```python
from build123d import *

# Parameters (mm, degrees)
SKETCH_3_W                      = 27
SKETCH_3_H                      = 27
EXTRUDE_1_DEPTH                 = 3
FILLET_1_R                      = 2
SKETCH_4_R                      = 1.1
CUT_EXTRUDE_1_DEPTH             = 6
SKETCH_5_R                      = 1.55
CUT_EXTRUDE_2_DEPTH             = 6
SKETCH_6_R                      = 1.05
CUT_EXTRUDE_3_DEPTH             = 6
PATTERN_CIRCULAR_1_COUNT        = 4
SKETCH_7_R                      = 4
CUT_EXTRUDE_4_DEPTH             = 1
CUT_EXTRUDE_8_DEPTH             = 21.012496096
PATTERN_CIRCULAR_2_COUNT        = 4
PATTERN_CIRCULAR_2_COPY_1_DEPTH = 21.012496096
PATTERN_CIRCULAR_2_COPY_2_DEPTH = 21.012496096
PATTERN_CIRCULAR_2_COPY_3_DEPTH = 21.012496096
SKETCH_12_R                     = 1.35
CUT_EXTRUDE_9_DEPTH             = 8
PATTERN_CIRCULAR_3_COUNT        = 4
EXTRUDE_2_DEPTH                 = 0.75
PATTERN_CIRCULAR_4_COUNT        = 4
PATTERN_CIRCULAR_4_COPY_1_DEPTH = 0.75
PATTERN_CIRCULAR_4_COPY_2_DEPTH = 0.75
PATTERN_CIRCULAR_4_COPY_3_DEPTH = 0.75
SKETCH_22_W                     = 2.7
SKETCH_22_H                     = 3
CUT_EXTRUDE_15_DEPTH            = 2
PATTERN_CIRCULAR_11_COUNT       = 4
SKETCH_31_W                     = 88
SKETCH_31_H                     = 100
EXTRUDE_4_DEPTH                 = 18
SKETCH_32_W                     = 78
SKETCH_32_H                     = 8.5
CUT_EXTRUDE_17_DEPTH            = 95


with BuildPart() as part:
    # ｽｹｯﾁ3 → ﾎﾞｽ - 押し出し1 (new, symmetric)
    with BuildSketch(Plane(origin=(0, 0, 0), x_dir=(1, 0, 0), z_dir=(0, 1, 0))):
        Rectangle(SKETCH_3_W, SKETCH_3_H)
    extrude(amount=EXTRUDE_1_DEPTH, both=True)

    # ﾌｨﾚｯﾄ1
    fillet_1_edges = [part.edges().sort_by_distance(p)[0] for p in [
        (13.5, 0, 13.5),
        (-13.5, 0, 13.5),
        (-13.5, 0, -13.5),
        (13.5, 0, -13.5),
    ]]
    fillet(fillet_1_edges, radius=FILLET_1_R)

    # ｽｹｯﾁ4 → ｶｯﾄ - 押し出し1 (cut)
    with BuildSketch(Plane(origin=(0, 3, 0), x_dir=(1, 0, 0), z_dir=(0, 1, 0))):
        with Locations(Location((-10.5, 10.5, 0), (0, 0, 270))):
            Circle(SKETCH_4_R)
        with Locations(Location((10.5, 10.5, 0), (0, 0, 270))):
            Circle(SKETCH_4_R)
        with Locations(Location((-10.5, -10.5, 0), (0, 0, 270))):
            Circle(SKETCH_4_R)
        with Locations(Location((10.5, -10.5, 0), (0, 0, 270))):
            Circle(SKETCH_4_R)
    extrude(amount=-CUT_EXTRUDE_1_DEPTH, mode=Mode.SUBTRACT)

    # ｽｹｯﾁ5 → ｶｯﾄ - 押し出し2 (cut)
    with BuildSketch(Plane(origin=(0, 3, 0), x_dir=(1, 0, 0), z_dir=(0, 1, 0))):
        with Locations(Location((0, 0, 0), (0, 0, 270))):
            Circle(SKETCH_5_R)
    extrude(amount=-CUT_EXTRUDE_2_DEPTH, mode=Mode.SUBTRACT)

    # ｽｹｯﾁ6 → ｶｯﾄ - 押し出し3 (cut)
    with BuildSketch(Plane(origin=(0, 3, 0), x_dir=(1, 0, 0), z_dir=(0, 1, 0))):
        with Locations(Location((4.242640687, 4.242640687, 0), (0, 0, 270))):
            Circle(SKETCH_6_R)
    cut_extrude_3 = extrude(amount=-CUT_EXTRUDE_3_DEPTH, mode=Mode.SUBTRACT)

    # 円形ﾊﾟﾀｰﾝ1: ｶｯﾄ - 押し出し3 ×4 about axis
    pattern_circular_1_axis = Axis((0, 0, 0), (0, 1, 0))
    for i in range(1, PATTERN_CIRCULAR_1_COUNT):
        add(cut_extrude_3.rotate(pattern_circular_1_axis, i * 360 / PATTERN_CIRCULAR_1_COUNT), mode=Mode.SUBTRACT)

    # ｽｹｯﾁ7 → ｶｯﾄ - 押し出し4 (cut)
    with BuildSketch(Plane(origin=(0, 3, 0), x_dir=(1, 0, 0), z_dir=(0, 1, 0))):
        with Locations(Location((0, 0, 0), (0, 0, 270))):
            Circle(SKETCH_7_R)
    extrude(amount=-CUT_EXTRUDE_4_DEPTH, mode=Mode.SUBTRACT)

    # ｽｹｯﾁ11 → ｶｯﾄ - 押し出し8 (cut, symmetric)
    with BuildSketch(Plane(origin=(0, 3, 0), x_dir=(1, 0, 0), z_dir=(0, 1, 0))):
        Polygon((-28.082033535, 86.024744916), (3, 13.5), (4.5, 10), (7, 10), (7.9, 13.5), (27.55047658, 89.918520033), (16.532211377, 247.342544779), (-39.100298738, 243.448769662), align=None)
    cut_extrude_8 = extrude(amount=CUT_EXTRUDE_8_DEPTH, both=True, mode=Mode.SUBTRACT)

    # ﾐﾗｰ1: ｶｯﾄ - 押し出し8 across plane
    add(cut_extrude_8.mirror(Plane(origin=(0, 0, 0), x_dir=(0, 0, 1), z_dir=(1, 0, 0))), mode=Mode.SUBTRACT)

    # 円形ﾊﾟﾀｰﾝ2: ｶｯﾄ - 押し出し8 ×4 about axis
    pattern_circular_2_axis = Axis((0, 0, 0), (0, 1, 0))
    for i in range(1, PATTERN_CIRCULAR_2_COUNT):
        add(cut_extrude_8.rotate(pattern_circular_2_axis, i * 360 / PATTERN_CIRCULAR_2_COUNT), mode=Mode.SUBTRACT)

    # 円形ﾊﾟﾀｰﾝ2 copy 1 sketch → 円形ﾊﾟﾀｰﾝ2 copy 1 (cut, symmetric)
    with BuildSketch(Plane.ZX.offset(3)):
        Polygon((-28.082033535, -86.024744916), (3, -13.5), (4.5, -10), (7, -10), (7.9, -13.5), (27.55047658, -89.918520033), (16.532211377, -247.342544779), (-39.100298738, -243.448769662), align=None)
    extrude(amount=PATTERN_CIRCULAR_2_COPY_1_DEPTH, both=True, mode=Mode.SUBTRACT)

    # 円形ﾊﾟﾀｰﾝ2 copy 2 sketch → 円形ﾊﾟﾀｰﾝ2 copy 2 (cut, symmetric)
    with BuildSketch(Plane(origin=(0, 3, 0), x_dir=(1, 0, 0), z_dir=(0, 1, 0))):
        Polygon((-28.082033535, -86.024744916), (3, -13.5), (4.5, -10), (7, -10), (7.9, -13.5), (27.55047658, -89.918520033), (16.532211377, -247.342544779), (-39.100298738, -243.448769662), align=None)
    extrude(amount=PATTERN_CIRCULAR_2_COPY_2_DEPTH, both=True, mode=Mode.SUBTRACT)

    # 円形ﾊﾟﾀｰﾝ2 copy 3 sketch → 円形ﾊﾟﾀｰﾝ2 copy 3 (cut, symmetric)
    with BuildSketch(Plane(origin=(0, 3, 0), x_dir=(0, 0, -1), z_dir=(0, 1, 0))):
        Polygon((-28.082033535, -86.024744916), (3, -13.5), (4.5, -10), (7, -10), (7.9, -13.5), (27.55047658, -89.918520033), (16.532211377, -247.342544779), (-39.100298738, -243.448769662), align=None)
    extrude(amount=PATTERN_CIRCULAR_2_COPY_3_DEPTH, both=True, mode=Mode.SUBTRACT)

    # ｽｹｯﾁ12 → ｶｯﾄ - 押し出し9 (cut)
    with BuildSketch(Plane.XY.offset(13.5)):
        Circle(SKETCH_12_R)
    cut_extrude_9 = extrude(amount=-CUT_EXTRUDE_9_DEPTH, mode=Mode.SUBTRACT)

    # 円形ﾊﾟﾀｰﾝ3: ｶｯﾄ - 押し出し9 ×4 about axis
    pattern_circular_3_axis = Axis((0, 0, 0), (0, 1, 0))
    for i in range(1, PATTERN_CIRCULAR_3_COUNT):
        add(cut_extrude_9.rotate(pattern_circular_3_axis, i * 360 / PATTERN_CIRCULAR_3_COUNT), mode=Mode.SUBTRACT)

    # ｽｹｯﾁ13 → ﾎﾞｽ - 押し出し2 (add, symmetric)
    with BuildSketch(Plane(origin=(0, 0, 0), x_dir=(1, 0, 0), z_dir=(0, 1, 0))):
        Polygon((7.9, 13.5), (7, 10), (6.5, 10), (7.4, 13.5), align=None)
        Polygon((3, 13.5), (3.5, 13.5), (5, 10), (4.5, 10), align=None)
    extrude_2 = extrude(amount=EXTRUDE_2_DEPTH, both=True)

    # ﾐﾗｰ2: ﾎﾞｽ - 押し出し2 across plane
    add(extrude_2.mirror(Plane(origin=(0, 0, 0), x_dir=(0, 0, 1), z_dir=(1, 0, 0))))

    # 円形ﾊﾟﾀｰﾝ4: ﾎﾞｽ - 押し出し2 ×4 about axis
    pattern_circular_4_axis = Axis((0, 0, 0), (0, 1, 0))
    for i in range(1, PATTERN_CIRCULAR_4_COUNT):
        add(extrude_2.rotate(pattern_circular_4_axis, i * 360 / PATTERN_CIRCULAR_4_COUNT))

    # 円形ﾊﾟﾀｰﾝ4 copy 1 sketch → 円形ﾊﾟﾀｰﾝ4 copy 1 (add, symmetric)
    with BuildSketch(Plane.ZX):
        Polygon((7.9, -13.5), (7, -10), (6.5, -10), (7.4, -13.5), align=None)
        Polygon((3, -13.5), (3.5, -13.5), (5, -10), (4.5, -10), align=None)
    extrude(amount=PATTERN_CIRCULAR_4_COPY_1_DEPTH, both=True)

    # 円形ﾊﾟﾀｰﾝ4 copy 2 sketch → 円形ﾊﾟﾀｰﾝ4 copy 2 (add, symmetric)
    with BuildSketch(Plane(origin=(0, 0, 0), x_dir=(1, 0, 0), z_dir=(0, 1, 0))):
        Polygon((7.9, -13.5), (7, -10), (6.5, -10), (7.4, -13.5), align=None)
        Polygon((3, -13.5), (3.5, -13.5), (5, -10), (4.5, -10), align=None)
    extrude(amount=PATTERN_CIRCULAR_4_COPY_2_DEPTH, both=True)

    # 円形ﾊﾟﾀｰﾝ4 copy 3 sketch → 円形ﾊﾟﾀｰﾝ4 copy 3 (add, symmetric)
    with BuildSketch(Plane(origin=(0, 0, 0), x_dir=(0, 0, -1), z_dir=(0, 1, 0))):
        Polygon((7.9, -13.5), (7, -10), (6.5, -10), (7.4, -13.5), align=None)
        Polygon((3, -13.5), (3.5, -13.5), (5, -10), (4.5, -10), align=None)
    extrude(amount=PATTERN_CIRCULAR_4_COPY_3_DEPTH, both=True)

    # ｽｹｯﾁ22 → ｶｯﾄ - 押し出し15 (cut)
    with BuildSketch(Plane.XY.offset(13.5)):
        with Locations((0, 1.5)):
            Rectangle(SKETCH_22_W, SKETCH_22_H)
    cut_extrude_15 = extrude(amount=-CUT_EXTRUDE_15_DEPTH, mode=Mode.SUBTRACT)

    # 円形ﾊﾟﾀｰﾝ11: ｶｯﾄ - 押し出し15 ×4 about axis
    pattern_circular_11_axis = Axis((0, 0, 0), (0, 1, 0))
    for i in range(1, PATTERN_CIRCULAR_11_COUNT):
        add(cut_extrude_15.rotate(pattern_circular_11_axis, i * 360 / PATTERN_CIRCULAR_11_COUNT), mode=Mode.SUBTRACT)

    # ｽｹｯﾁ31 → ﾎﾞｽ - 押し出し4 (add)
    with BuildSketch(Plane.XZ.offset(3)):
        with Locations((0, -20)):
            Rectangle(SKETCH_31_W, SKETCH_31_H)
    extrude(amount=EXTRUDE_4_DEPTH)

    # ｽｹｯﾁ32 → ｶｯﾄ - 押し出し17 (cut)
    with BuildSketch(Plane.XY.offset(30)):
        with Locations((0, -11.75)):
            Rectangle(SKETCH_32_W, SKETCH_32_H)
    extrude(amount=-CUT_EXTRUDE_17_DEPTH, mode=Mode.SUBTRACT)


solid = part.part
```
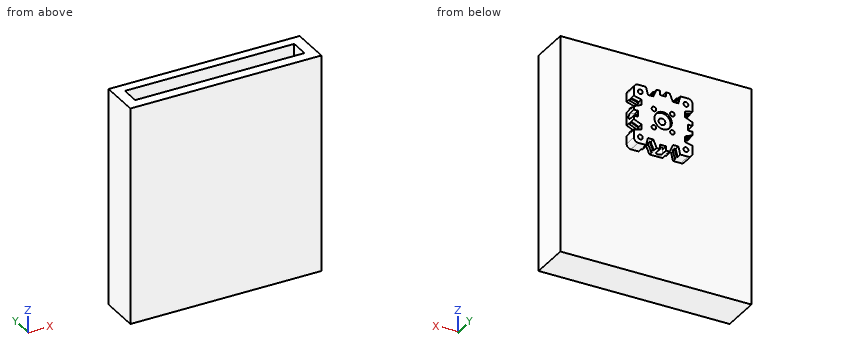
Design review of the part built by this model. Coordinates are the model's own, in mm. Give positions to 0.01 mm unless a question says otherwise; leave off trailing zeros. Write each loop counter-clockwise with the first axis right and the second up, starting at its lowest first coordinate (ties: lowest second). Pieces come first, ordered by that corner, then holes. Notation, with made-up numbers: (-32.75, -3.5) - (-24.75, -3.5) arc R22 ccw to (-24.75, 3.5) - close; hole circle Ø3 at (49, -3). An arc over 180 degrees is marked (long way). Return JSON: item names as keys, results as strings. Group by question number.
(1) We need section A-A, the plane z = 0. Give the boundary of the cut face in (x, y).
(2) We need section C-C, the plane y = -10. Give the boundary of the cut face in (x, z), then the cut area to 3 significant figures.
(3) Insertion check: pin 1 (1.6 mm diameter, centred on y = 2, z = -13, fed in from +X); pin 2 (3 mm diameter, centred on x = -1, y = -1, fed in from +Z); pin 3 (1.6 mm diameter, centred on x = 13, y = 2, fed in from +Z). Each pin has a flat end and moves straight along its axis. Give the tip position at first contact, or say it passes through.
(4) We need section D-D, the plane x = -22. Give the boundary of the cut face in (y, z).
(5) To check wall thickness, follow probe 1 along Y at (x, z) = (-3, -20); probe 2 along Z at (x, y) = (-10.75, 0); probe 3 along X at (y, z) = (-14.5, -64.5). State the ranges of each line that lie inside material, in increasing order.
(6) We need section B-B, the plane x = 0. Give the boundary of the cut face in (y, z), then the cut area to 3 significant figures.
Reported:
{
 "1": {"outline": "(-44, -21) - (44, -21) - (44, -3) - (13.5, -3) - (13.5, -1.35) - (5.5, -1.35) - (5.5, 1.35) - (11.5, 1.35) - (11.5, 3) - (4, 3) - (4, 2) - (1.55, 2) - (1.55, -3) - (-1.55, -3) - (-1.55, 2) - (-4, 2) - (-4, 3) - (-11.5, 3) - (-11.5, 1.35) - (-5.5, 1.35) - (-5.5, -1.35) - (-13.5, -1.35) - (-13.5, -3) - (-44, -3) - close; hole (-39, -16) - (39, -16) - (39, -7.5) - (-39, -7.5) - close"},
 "2": {"outline": "(-44, -70) - (44, -70) - (44, 30) - (39, 30) - (39, -65) - (-39, -65) - (-39, 30) - (-44, 30) - close", "area": "1,390 mm2"},
 "3": {"pin 1": "stops at x = 13.37", "pin 2": "stops at z = 13.5", "pin 3": "stops at z = 13.37"},
 "4": {"outline": "(-21, -70) - (-3, -70) - (-3, 30) - (-7.5, 30) - (-7.5, -65) - (-16, -65) - (-16, 30) - (-21, 30) - close"},
 "5": {"probe 1": "y = -21 to -16, -7.5 to -3", "probe 2": "z = -13.5 to -11.57, -9.43 to -6.69, -4.68 to -1.35, 1.35 to 4.68, 6.69 to 9.43, 11.57 to 13.5", "probe 3": "x = -44 to -39, 39 to 44"},
 "6": {"outline": "(-21, -70) - (-3, -70) - (-3, -13.5) - (-1.35, -13.5) - (-1.35, -5.5) - (1.35, -5.5) - (1.35, -11.5) - (3, -11.5) - (3, -4) - (2, -4) - (2, -1.55) - (-3, -1.55) - (-3, 1.55) - (2, 1.55) - (2, 4) - (3, 4) - (3, 11.5) - (1.35, 11.5) - (1.35, 5.5) - (-1.35, 5.5) - (-1.35, 13.5) - (-3, 13.5) - (-3, 30) - (-7.5, 30) - (-7.5, -65) - (-16, -65) - (-16, 30) - (-21, 30) - close", "area": "1,080 mm2"}
}
